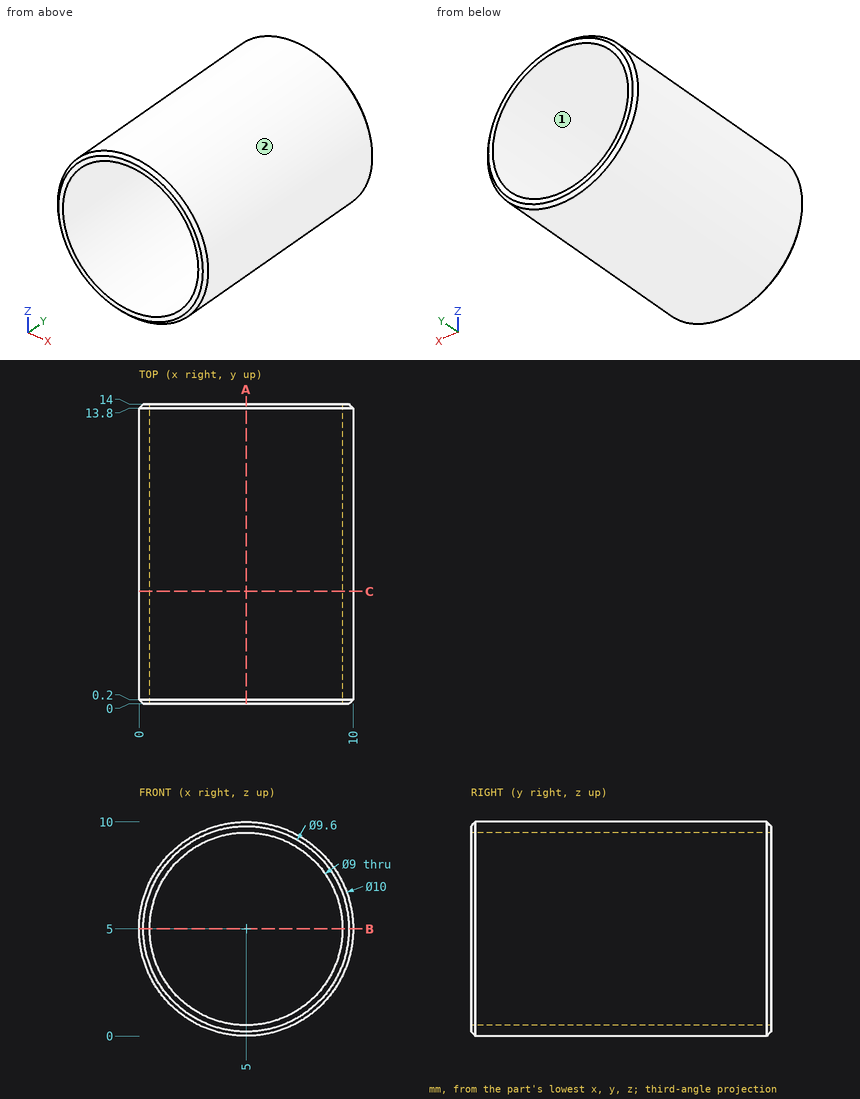
Geometry check sheet. Reference: drawing and pictorial views, mm from the part's lowest x, y, z. Coordinates: 2 decimals unless noted, no trailing zeros. Order: outer loops, then holes, each group sorted by start corner. A loop starts at its lowest first (then second) coordinate and runs counter-clockwise, first axis right, second up. Notation, with made-up numbers: (46, 8) -> (71, 8) arc R27 ccw to (71, 36) -> close; hole circle Ø6 at (75, 81). An arc over 180 degrees is marked (long way). Write item = value, one per line. Start each with the question number.
1) Mould release check, pull along X, two halves, no side actions. Record for the marked faces 1 and 2: +X half, -X half, draft (parallel to the pull), parting line (faces both ways), or undercut.
2) Material ranges on L1, parallel to Z at x = 5, y = 7.5; L2, parallel to Z at x = 4, y = 8.5; L3, parallel to X at y = 9, z = 3.75, recorded low to high.
3) Cross-section at A-A (x = 5). Enter the section's corners in (y, z), then the cut area to 3 significant figures.
4) Cross-section at C-C (y = 5.25). Enter the section's corners in (x, z), then the cut area to 3 significant figures.
5) Go/stop test with flat-tipped pins: P1, Ø1.5, axis at x = 4, y = 10.5, coming from the +Z side; P2, Ø3, axis at x = 2, y = 11, coming from the +Z side; P3, Ø1, axis at x = 7.5, z = 2, coming from the -Y side; P4, Ø2, axis at y = 4, z = 8.5, coming from the -X side. Record where each tip stops, or that it passes through.
6) Cross-section at B-B (z = 5). Enter the section's corners in (x, y).
Ans:
q1.face_1 = undercut
q1.face_2 = parting line
q2.L1 = 0 to 0.5, 9.5 to 10
q2.L2 = 0.1 to 0.61, 9.39 to 9.9
q2.L3 = 0.16 to 0.68, 9.32 to 9.84
q3.outline = (0, 0.2) -> (0.2, 0) -> (13.8, 0) -> (14, 0.2) -> (14, 0.5) -> (0, 0.5) -> close; (0, 9.5) -> (14, 9.5) -> (14, 9.8) -> (13.8, 10) -> (0.2, 10) -> (0, 9.8) -> close
q3.area = 13.9 mm²
q4.outline = circle Ø10 at (5, 5); hole circle Ø9 at (5, 5)
q4.area = 14.9 mm²
q5.P1 = 9.99
q5.P2 = 9.77
q5.P3 = through
q5.P4 = 0.67
q6.outline = (0, 0.2) -> (0.2, 0) -> (0.5, 0) -> (0.5, 14) -> (0.2, 14) -> (0, 13.8) -> close; (9.5, 0) -> (9.8, 0) -> (10, 0.2) -> (10, 13.8) -> (9.8, 14) -> (9.5, 14) -> close
